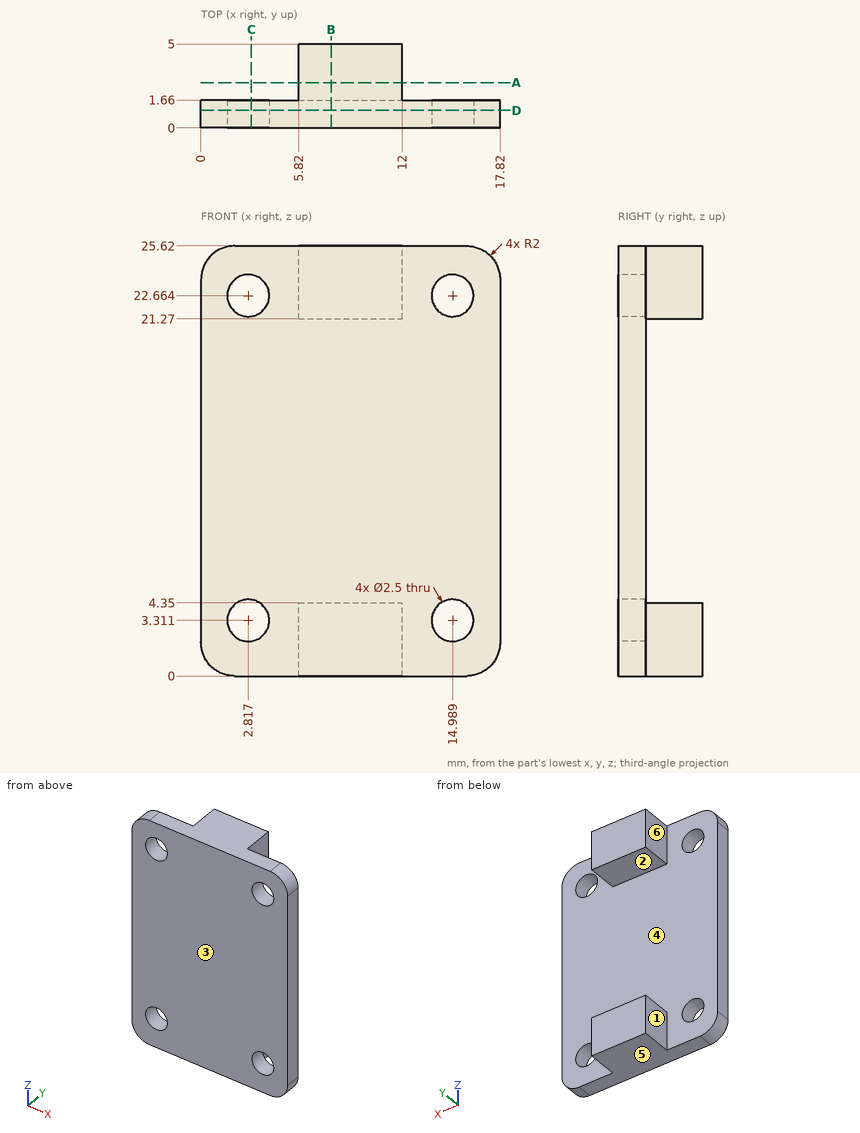
Part print with two shaded views. Sizes in mm from the minimum x, y, z corner. A direction names the side the tool comes from. Coordinates: 2 decimals unless noted, no trailing zeros. Order: outer loops, then holes, each group sorted by start corner. A loop starts at its lowest first (then second) coordinate and runs counter-clockwise, first axis right, second up. Notation, with made-up numbers: M 17.25,-8 L 33.25,-8 A31 ccw 33.25,21 Z; hole C 86,47 d10. An arc over 180 degrees is marked long. One line per question, with ' | ' between items. Start each with the question number.
1. Cut at D-D (y = 1.05). Write the cut outline in (x, z).
2. Cut at B-B (x = 7.75). Write the cut outline in (y, z).
3. Tool access for the marked faces 1, 2 and 3: list every direction of +Z, -Z, +X, -X, +Y, -Y with a clear straight run to the whole face (end or side of a thin tool).
4. Wall check: line 1 along Z through (x, y) = (7, 3.2); line 2 along Y through (x, z) = (9.5, 9); line 3 along X through (y, z) = (1.95, 3.75). Give the ranges that are in metal, low to high. Write a range as [from, to].
5. Mould opens along Z. For the marked faces 4, 5 and 6 say: +Z half, -Z half, draft (parallel to the pull), parting line (faces both ways), or undercut.
6. Cut at A-A (y = 2.7). Write the cut outline in (x, z).
7. Cut at C-C (x = 3). Write the cut outline in (y, z), plus the area to 3 significant figures.
8. Flat gauge pins, fed straight in: P1, Ø3, axis at x = 14.99, z = 22.66, coming from the +Y side; P2, Ø2, axis at x = 10, y = 2.5, coming from the -Z side; P3, Ø1, axis at y = 3.5, z = 23.5, coming from the +X side; P4, Ø1.7, axis at y = 3.5, z = 3, coming from the -X side. Where does each tip first touch, or does it go through?
The answers:
1) outline: M 0,2 A2 ccw 2,0 L 15.82,0 A2 ccw 17.82,2 L 17.82,23.62 A2 ccw 15.82,25.62 L 2,25.62 A2 ccw 0,23.62 Z; hole C 2.82,3.31 d2.5; hole C 2.82,22.66 d2.5; hole C 14.99,3.31 d2.5; hole C 14.99,22.66 d2.5
2) outline: M 0,0 L 5,0 L 5,4.35 L 1.66,4.35 L 1.66,21.27 L 5,21.27 L 5,25.62 L 0,25.62 Z
3) face 1: +Z, -Z, -X, +Y | face 2: +X, -X, +Y | face 3: +Z, -Z, +X, -X, -Y
4) line 1: z = [0, 4.35], [21.27, 25.62] | line 2: y = [0, 1.66] | line 3: x = [5.82, 12]
5) face 4: undercut | face 5: -Z half | face 6: draft
6) outline: M 5.82,0 L 12,0 L 12,4.35 L 5.82,4.35 Z; M 5.82,21.27 L 12,21.27 L 12,25.62 L 5.82,25.62 Z
7) outline: M 0,0 L 1.66,0 L 1.66,2.07 L 0,2.07 Z; M 0,4.55 L 1.66,4.55 L 1.66,21.43 L 0,21.43 Z; M 0,23.9 L 1.66,23.9 L 1.66,25.62 L 0,25.62 Z | area: 34.3 mm2
8) P1: stops at y = 1.66 | P2: stops at z = 0 | P3: stops at x = 12 | P4: stops at x = 5.82
